from build123d import *

# Parameters (mm, degrees)
SKETCH_1_R          = 5
EXTRUDE_1_DEPTH     = 5
SKETCH_1_3_W        = 15
SKETCH_1_3_H        = 5
SKETCH_1_3_H_2      = 15
EXTRUDE_2_DEPTH     = 15
CUT_EXTRUDE_1_DEPTH = 15
CUT_EXTRUDE_2_DEPTH = 10
SCALE_1_SCALE       = 0.2


with BuildPart() as part:
    # Sketch 1 → Extrude 1 (new body)
    with BuildSketch(Plane(origin=(0, 0, 0), x_dir=(1, 0, 0), z_dir=(0, 1, 0))):
        with BuildLine():
            ThreePointArc((0, -10), (10, 0), (0, 10))
            Line((0, 10), (-10, 10))
            Line((-10, 10), (-10, 5))
            Line((-10, 5), (-10, -10))
            Line((-10, -10), (0, -10))
        make_face()
        Circle(SKETCH_1_R, mode=Mode.SUBTRACT)
    extrude(amount=EXTRUDE_1_DEPTH)

    # Sketch 1_3 → Extrude 2 (add)
    with BuildSketch(Plane(origin=(0, 0, 0), x_dir=(1, 0, 0), z_dir=(0, 1, 0))):
        with Locations((-17.5, 7.5)):
            Rectangle(SKETCH_1_3_W, SKETCH_1_3_H)
        with Locations((-17.5, -2.5)):
            Rectangle(SKETCH_1_3_W, SKETCH_1_3_H_2)
    extrude(amount=EXTRUDE_2_DEPTH)

    # Sketch 3 → Cut-Extrude 1 (cut)
    with BuildSketch(Plane(origin=(-10, 0, 0), x_dir=(0, 0, -1), z_dir=(1, 0, 0))):
        Polygon((5, 15), (-10, 10), (-10, 15), align=None)
    extrude(amount=-CUT_EXTRUDE_1_DEPTH, mode=Mode.SUBTRACT)

    # Sketch 2 → Cut-Extrude 2 (cut)
    with BuildSketch(Plane(origin=(0, 15, 0), x_dir=(1, 0, 0), z_dir=(0, 1, 0))):
        Polygon((-10, 5), (-20, -10), (-10, -10), align=None)
    extrude(amount=-CUT_EXTRUDE_2_DEPTH, mode=Mode.SUBTRACT)


with BuildPart() as part_1:
    # Scale 1: scaled about (-13.252128035, 5.281976431, -1.035154021)
    add(part.part.scale(SCALE_1_SCALE).moved(Location((-10.601702428, 4.225581145, -0.828123217))))


solid = part_1.part
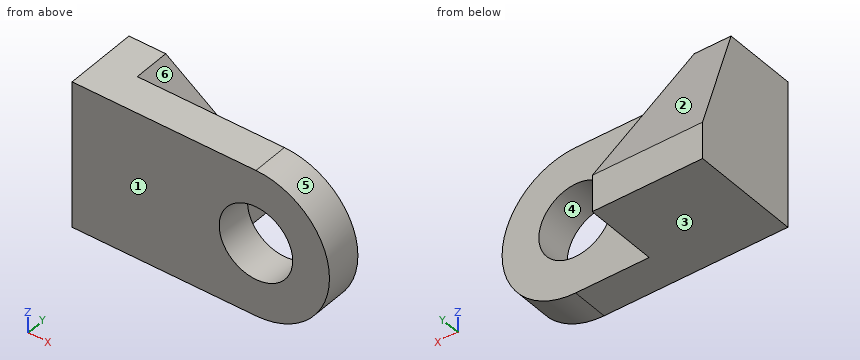
Here's how the part is built. I have some questions about the finished solid (model axes, mm). Face numbers are marked on the shaded views. A direction names the side the tool comes from. Give positions to 0.01 mm unless a question says otherwise; leave off trailing zeros. Order: outer loops, then holes, each group sorted by start corner. A loop starts at its lowest first (then second) coordinate and runs counter-clockwise, first axis right, second up. Notation, with made-up numbers: M 25,-25 L 51,-25 A14 ccw 51,-10 Z; hole C -19.75,66.25 d2. An arc over 180 degrees is marked long. Answer as a JSON object with one key per item and string values. Group by question number.
1) Suppose I cut it at C-C, the plane y = 4.8. Write out the boundary of the cut face in (x, z).
2) Suppose I cut it at B-B, the plane x = -10.5. Write out the boundary of the cut face in (y, z), plus the area to 3 significant figures.
3) Please list where these lines run through material, in increasing order: L1, parallel to Y at x = -13, z = -0.45; L2, parallel to X at y = 6.85, z = -2.2; L3, parallel to Z at x = -9.75, y = 4.7. Write a range as [from, to].
4) Suppose I cut it at D-D, the plane y = 5.55. Write out the boundary of the cut face in (x, z), plus the area to 3 significant figures.
5) I'm going to push a flat-ended pin straight in: pin 1 Ø0.8 at (y, z) = (6, -2.5) entering from +X. Where does the tip first touch, or does it pass through?
6) On a 3-axis mill with a long thin cutter (end or side, diameter ignored), from which of +Z, -Z, +X, -X, +Y, -Y can I reach the whole of each face in a straight line? I mean the marked faces 5 and 6. Say none if no direction works.
7) We'd pull the mould along Z, two halves only. Please class the marked faces 1, 2, 3 and 4: pulls with the +Z half, pulls with the -Z half, needs draft (parallel to the pull), parting line crosses it, or undercut.
8) Suppose I cut it at A-A, the plane z = -1. Write out the boundary of the cut face in (x, y).
Results found:
{
 "1": {"outline": "M -15.6,-2.83 L -10.6,-2.83 A2 ccw -10.6,1.17 L -15.6,1.17 Z; hole C -10.6,-0.83 d2"},
 "2": {"outline": "M 4.23,-2.83 L 5.23,-2.83 L 5.23,-1.82 L 4.23,-1.82 Z; M 4.23,0.17 L 5.23,0.17 L 5.23,1.17 L 4.23,1.17 Z", "area": "2.01 mm²"},
 "3": {"L1": "[4.23, 5.23]", "L2": "[-15.6, -12.6]", "L3": "[-2.64, -1.35], [-0.3, 0.98]"},
 "4": {"outline": "M -15.6,-2.83 L -12.6,-2.83 L -12.6,-1.83 L -14.6,1.17 L -15.6,1.17 Z", "area": "9.00 mm²"},
 "5": {"pin 1": "x = -12.6"},
 "6": {"face 5": "+X, +Y, -Y", "face 6": "+Z, +X, +Y"},
 "7": {"face 1": "needs draft", "face 2": "pulls with the +Z half", "face 3": "pulls with the -Z half", "face 4": "undercut"},
 "8": {"outline": "M -15.6,4.23 L -11.59,4.23 L -11.59,5.23 L -13.15,5.23 L -13.15,6.95 L -15.6,6.95 Z; M -9.62,4.23 L -8.61,4.23 L -8.61,5.23 L -9.62,5.23 Z"}
}
